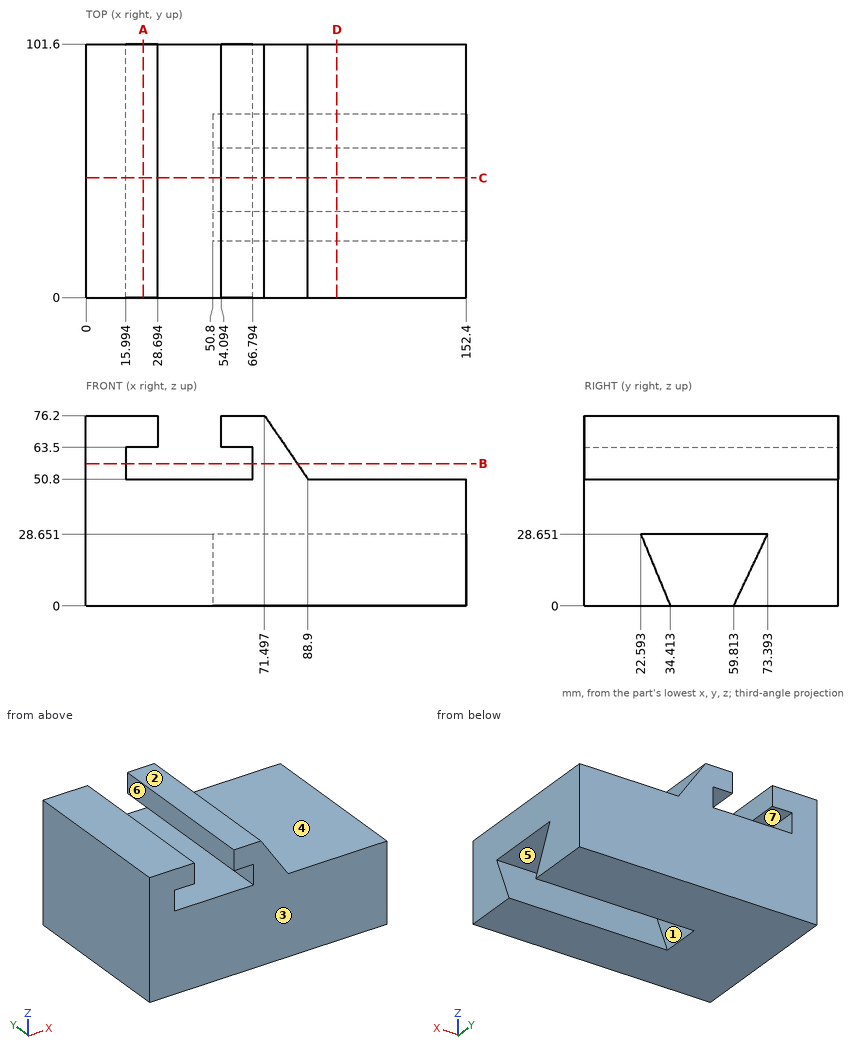
Input: dimensioned drawing with shaded views. Units: mm. Origin: part minimum x, y, z. A direction names the side the tool comes from. Round coordinates to 2 decimals unless told otherwise and drop trailing zeros. Loops run counter-clockwise (first coordinate to the right, second up) from the corner with the lowest first, then second, coordinate; pieces in that order, holes last.
1) Section query C-C on y = 48. Return the cut outline in (x, z), plus the area to 3 significant figures.
Ans:
outline: (0, 0) - (50.8, 0) - (50.8, 28.65) - (152.4, 28.65) - (152.4, 50.8) - (88.9, 50.8) - (71.5, 76.2) - (54.09, 76.2) - (54.09, 63.5) - (66.79, 63.5) - (66.79, 50.8) - (15.99, 50.8) - (15.99, 63.5) - (28.69, 63.5) - (28.69, 76.2) - (0, 76.2) - close
area: 5,900 mm2
2) Material intervals for line 1 (Z direction, x = 62, y = 85); line 2 (Z direction, x = 128, y = 9.5); line 3 (X direction, y = 58.5, z = 65) (1 decimal), sorted ascending.
Ans:
line 1: z = 0 to 50.8, 63.5 to 76.2
line 2: z = 0 to 50.8
line 3: x = 0 to 28.7, 54.1 to 79.2
3) Pull-direction query (Y, two-part tool) for the marked faces 1, 2 and 3; classes: released by +Y, released by -Y, zero draft, split by the parting line, or undercut.
Ans:
face 1: undercut
face 2: zero draft
face 3: released by -Y
4) Section query D-D on x = 100.5. Return the cut outline in (y, z).
Ans:
outline: (0, 0) - (34.41, 0) - (22.59, 28.65) - (73.39, 28.65) - (59.81, 0) - (101.6, 0) - (101.6, 50.8) - (0, 50.8) - close
5) Section query A-A on x = 23. Return the cut outline in (y, z), plus the area to 3 significant figures.
Ans:
outline: (0, 0) - (101.6, 0) - (101.6, 50.8) - (0, 50.8) - close; (0, 63.5) - (101.6, 63.5) - (101.6, 76.2) - (0, 76.2) - close
area: 6,450 mm2
6) Section query B-B on z = 57. Return the cut outline in (x, y), plus the area to 3 significant figures.
Ans:
outline: (0, 0) - (15.99, 0) - (15.99, 101.6) - (0, 101.6) - close; (66.79, 0) - (84.65, 0) - (84.65, 101.6) - (66.79, 101.6) - close
area: 3,440 mm2
7) Set-up query: the marked faces 4, 5, 6 and 7. Return all of +Z, -Z, +X, -X, +Y, -Y with unobstructed straight access to the full face (end or side cutting, diameter ignored); none if empty.
Ans:
face 4: +Z, +X, +Y, -Y
face 5: +X
face 6: +Z, +Y, -Y
face 7: +Y, -Y
8) Pin query (flat end, axial travel): pin 1 (10 mm diameter, centred on y = 69, z = 59, fed in from +X); pin 2 (8 mm diameter, centred on x = 71.5, y = 45, fed in from -Z); pin 3 (3 mm diameter, centred on x = 124.5, y = 36.5, fed in from +Z). Return the tip coordinate at first contact, or that it passes through.
Ans:
pin 1: stops at x = 86.71
pin 2: stops at z = 28.65
pin 3: stops at z = 50.8
